Source: CAD feature listing. Evaluate the final solid. Frame: model axes, mm. Coordinates: 2 decimals unless noted, no trailing zeros. Write each loop counter-clockwise with the first axis right and the second up, starting at its lowest first coordinate (ties: lowest second). Pieces come first, ordered by that corner, then holes. Notation, with made-up numbers: (46.5, -12.75) -> (60.5, -12.75) arc R8 ccw to (60.5, -8.75) -> close; hole circle Ø9 at (70, -26). An arc over 180 degrees is marked (long way). Write item = value, one per line.
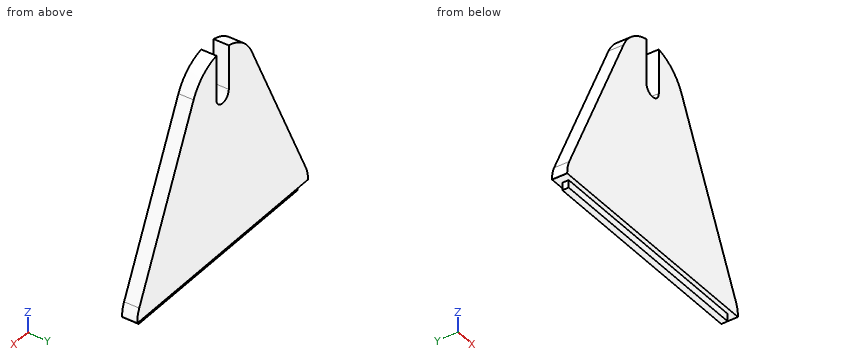
from build123d import *

# Parameters (mm, degrees)
BOSS_EXTRUDE1_DEPTH = 5
SKETCH3_W           = 80
SKETCH3_H           = 5
BOSS_EXTRUDE2_DEPTH = 5
SKETCH6_W           = 80
SKETCH6_H           = 5
SKETCH6_W_2         = 74.5
SKETCH6_H_2         = 2.1
CUT_EXTRUDE2_DEPTH  = 2.5
FILLET1_R           = 10
CUT_EXTRUDE3_DEPTH  = 5


with BuildPart() as part:
    # Sketch2 → Boss-Extrude1 (new body)
    with BuildSketch(Plane(origin=(0, 0, 0), x_dir=(1, 0, 0), z_dir=(0, 1, 0))):
        with BuildLine():
            Line((-40, 0), (40, 0))
            Line((40, 0), (13.582225242, -56.365780194))
            ThreePointArc((13.582225242, -56.365780194), (0, -65), (-13.582225242, -56.365780194))
            Line((-13.582225242, -56.365780194), (-40, 0))
        make_face()
    extrude(amount=BOSS_EXTRUDE1_DEPTH)

    # Sketch3 → Boss-Extrude2 (add)
    with BuildSketch(Plane(origin=(0, 0, 0), x_dir=(-1, 0, 0), z_dir=(0, 0, -1))):
        with Locations((0, 2.5)):
            Rectangle(SKETCH3_W, SKETCH3_H)
    extrude(amount=BOSS_EXTRUDE2_DEPTH)

    # Sketch6 → Cut-Extrude2 (cut)
    with BuildSketch(Plane(origin=(0, 0, -5), x_dir=(-1, 0, 0), z_dir=(0, 0, -1))):
        with Locations((0, 2.5)):
            Rectangle(SKETCH6_W, SKETCH6_H)
        with Locations((0, 2.5)):
            Rectangle(SKETCH6_W_2, SKETCH6_H_2, mode=Mode.SUBTRACT)
    extrude(amount=-CUT_EXTRUDE2_DEPTH, mode=Mode.SUBTRACT)

    # Fillet1
    fillet1_edges = [part.edges().sort_by_distance(p)[0] for p in [
        (-40, 2.5, 0),
        (40, 2.5, 0),
    ]]
    fillet(fillet1_edges, radius=FILLET1_R)

    # Sketch7 → Cut-Extrude3 (cut)
    with BuildSketch(Plane(origin=(0, 0, 0), x_dir=(-1, 0, 0), z_dir=(0, -1, 0))):
        with BuildLine():
            Line((2.9, -50), (2.9, -64.716996976))
            ThreePointArc((2.9, -64.716996976), (0, -65), (-2.9, -64.716996976))
            Line((-2.9, -64.716996976), (-2.9, -50))
            ThreePointArc((-2.9, -50), (0, -47.1), (2.9, -50))
        make_face()
    extrude(amount=-CUT_EXTRUDE3_DEPTH, mode=Mode.SUBTRACT)


solid = part.part
1) Cut plane D-D, the plane x = -11. Output: boundary loops of the cut face in (y, z), and give its area (3 significant figures).
Answer block:
outline = (0, -2.5) -> (1.45, -2.5) -> (1.45, -5) -> (3.55, -5) -> (3.55, -2.5) -> (5, -2.5) -> (5, 60.2) -> (0, 60.2) -> close
area = 319 mm2
2) Cut plane A-A, the plane y = 2.4. Output: boundary loops of the cut face in (x, z), and give its area (3 significant figures).
Answer block:
outline = (-40, -2.5) -> (-37.25, -2.5) -> (-37.25, -5) -> (37.25, -5) -> (37.25, -2.5) -> (40, -2.5) -> (40, -2.23) arc R10 ccw to (39.05, 2.02) -> (13.58, 56.37) arc R15 ccw to (2.9, 64.72) -> (2.9, 50) arc R2.9 cw to (-2.9, 50) -> (-2.9, 64.72) arc R15 ccw to (-13.58, 56.37) -> (-39.05, 2.02) arc R10 ccw to (-40, -2.23) -> close
area = 3,470 mm2
3) Cut plane B-B, the plane z = 52. Output: boundary loops of the cut face in (x, y), and give its area (3 significant figures).
Answer block:
outline = (-15.63, 0) -> (-2.9, 0) -> (-2.9, 5) -> (-15.63, 5) -> close; (2.9, 0) -> (15.63, 0) -> (15.63, 5) -> (2.9, 5) -> close
area = 127 mm2
4) First-contact query: pin 1 Ø1.5 at (x, y) = (20.5, 3.5) entering from +Z; pin 2 Ø2.5 at (y, z) = (2.5, 56.5) entering from -X; pin 3 Ø3 at (y, z) = (1, 3.5) entering from -X. Flat tips, straight axial feed; report the tip coordinate or a pass-through.
Answer block:
pin_1 = 43.21
pin_2 = -14.11
pin_3 = -39.06
5) Cut plane C-C, the plane x = 0. Output: boundary loops of the cut face in (y, z).
Answer block:
outline = (0, -2.5) -> (1.45, -2.5) -> (1.45, -5) -> (3.55, -5) -> (3.55, -2.5) -> (5, -2.5) -> (5, 47.1) -> (0, 47.1) -> close
6) Material intervals for probe 1 along X at (y, z) = (1.25, 58.5); probe 2 along Z at (x, y) = (-3, 1.8); probe 3 along X at (y, z) = (4.3, 16.5), sorted ascending. Write a range as [from, to].
Answer block:
probe_1 = [-12.36, -2.9], [2.9, 12.36]
probe_2 = [-5, 64.7]
probe_3 = [-32.27, 32.27]
